For this review, take the finished solid that the model builds, in its own axes (mm). A direction names the side the tool comes from. Coordinates: 2 decimals unless noted, no trailing zeros. Loops run counter-clockwise (first coordinate to the right, second up) from the corner with the lowest first, then second, coordinate; pieces in that order, holes last. Notation, with made-up numbers: (48, 55) -> (103, 55) arc R24 ccw to (103, 86) -> close; hole circle Ø11 at (11.25, 42.5). An arc over 180 degrees is marked (long way). One line per item, written item: value.
from build123d import *

# Parameters (mm, degrees)
SKETCH1_W             = 38.1
SKETCH1_H             = 38.1
BOSS_EXTRUDE1_DEPTH   = 6.35
BOSS_EXTRUDE2_DEPTH   = 38.1
CUT_EXTRUDE1_DEPTH    = 39.1
F_4_CLEARANCE_HOLE1_D = 3.4544
SKETCH6_R             = 3.96875
CUT_EXTRUDE2_DEPTH    = 6.35


with BuildPart() as part:
    # Sketch1 → Boss-Extrude1 (new body)
    with BuildSketch(Plane(origin=(0, 0, 0), x_dir=(1, 0, 0), z_dir=(0, 1, 0))):
        Rectangle(SKETCH1_W, SKETCH1_H)
    extrude(amount=BOSS_EXTRUDE1_DEPTH)

    # Sketch2 → Boss-Extrude2 (add)
    with BuildSketch(Plane.XY.offset(19.05)):
        with BuildLine():
            Line((-19.05, 6.35), (19.05, 6.35))
            ThreePointArc((19.05, 6.35), (10.069743762, 10.06974368), (6.349999801, 19.049999801))
            Line((6.349999801, 19.049999801), (-6.350000199, 19.049999801))
            ThreePointArc((-6.350000199, 19.049999801), (-10.06974402, 10.069743821), (-19.05, 6.35))
        make_face()
    extrude(amount=-BOSS_EXTRUDE2_DEPTH)

    # Sketch3 → Cut-Extrude1 (cut, through all)
    with BuildSketch(Plane(origin=(19.05, 0, 0), x_dir=(0, 0, -1), z_dir=(1, 0, 0))):
        with BuildLine():
            Line((-19.05, 6.35), (-19.05, 19.049999801))
            Line((-19.05, 19.049999801), (-6.350000199, 19.049999801))
            ThreePointArc((-6.350000199, 19.049999801), (-10.06974402, 10.069743821), (-19.05, 6.35))
        make_face()
        with BuildLine():
            Line((19.05, 6.35), (19.05, 19.049999801))
            Line((19.05, 19.049999801), (6.350000199, 19.049999801))
            ThreePointArc((6.350000199, 19.049999801), (10.06974402, 10.069743821), (19.05, 6.35))
        make_face()
    extrude(amount=-CUT_EXTRUDE1_DEPTH, mode=Mode.SUBTRACT)

    # #4 Clearance Hole1 (through all)
    with Locations(Plane(origin=(0, 19.049999801, 0), x_dir=(1, 0, 0), z_dir=(0, 1, 0))):
        with Locations((0, 0)):
            Hole(F_4_CLEARANCE_HOLE1_D / 2)

    # Sketch6 → Cut-Extrude2 (cut)
    with BuildSketch(Plane.XZ):
        Circle(SKETCH6_R)
    extrude(amount=-CUT_EXTRUDE2_DEPTH, mode=Mode.SUBTRACT)


solid = part.part
1. Take a section at C-C, the plane y = 4. Give the boundary of the cut face in (x, z).
Return value:
outline: (-19.05, -19.05) -> (19.05, -19.05) -> (19.05, 19.05) -> (-19.05, 19.05) -> close; hole circle Ø7.94 at (0, 0)
2. Insertion check: pin 1 Ø6 at (x, z) = (-13.5, -11.5) entering from +Y; pin 2 Ø6 at (x, y) = (2, 16.5) entering from +Z; pin 3 Ø10 at (x, y) = (9, 12.5) entering from -Z. Each pin has a flat end and moves straight along its axis. Give the tip position at first contact, or say it passes through.
Return value:
pin 1: stops at y = 9.54
pin 2: stops at z = 7.63
pin 3: stops at z = -13.77
3. To check wall thickness, follow probe 1 along Z at (x, y) = (1, 14.75); probe 2 along Z at (x, y) = (0, 11.25); probe 3 along X at (y, z) = (12.75, 2). State the ranges of each line that lie inside material, in increasing order. Write a range as from..to.
Return value:
probe 1: z = -7.1..-1.41, 1.41..7.1
probe 2: z = -9.03..-1.73, 1.73..9.03
probe 3: x = -8.02..8.02
4. For faces 5 (the cylindrical face through (-0.86, 3.131, -3.874)), 6 (the cylindrical face through (-11.65, 8.73, 0.27)), list the 3-axis set-ups (+Z, -Z, +X, -X, +Y, -Y) from which the entire face can be reached by the end or side of a thin tool; tool diameter is ignored.
Return value:
face 5: -Y
face 6: +Z, -Z, -X, +Y
5. Take a section at A-A, the plane x = 0. Give the boundary of the cut face in (y, z), and give its area (3 significant figures).
Return value:
outline: (0, -19.05) -> (6.35, -19.05) arc R12.7 cw to (19.05, -6.35) -> (19.05, -1.73) -> (6.35, -1.73) -> (6.35, -3.97) -> (0, -3.97) -> close; (0, 3.97) -> (6.35, 3.97) -> (6.35, 1.73) -> (19.05, 1.73) -> (19.05, 6.35) arc R12.7 cw to (6.35, 19.05) -> (0, 19.05) -> close
area: 378 mm2
6. Take a section at D-D, the plane z = -12. Give the boundary of the cut face in (x, y).
Return value:
outline: (-19.05, 0) -> (19.05, 0) -> (19.05, 6.35) arc R12.7 cw to (12, 8.49) -> (-12, 8.49) arc R12.7 cw to (-19.05, 6.35) -> close
7. The part is to be moulded in two halves that separate along Z. For faces 1 (the flat face through (-19.05, 3, 0)), 2 (the flat face through (2, 6.35, -1)), 3 (the cylindrical face through (0.27, 8.73, 11.65)), 4 (the cylindrical face through (0.27, 8.73, -11.65)), say which applies: pulls with the +Z half, pulls with the -Z half, needs draft (parallel to the pull), parting line crosses it, or undercut.
Return value:
face 1: needs draft
face 2: undercut
face 3: pulls with the +Z half
face 4: pulls with the -Z half
8. Take a section at B-B, the plane z = 0. Give the boundary of the cut face in (x, y).
Return value:
outline: (-19.05, 0) -> (-3.97, 0) -> (-3.97, 6.35) -> (-1.73, 6.35) -> (-1.73, 19.05) -> (-6.35, 19.05) arc R12.7 cw to (-19.05, 6.35) -> close; (1.73, 6.35) -> (3.97, 6.35) -> (3.97, 0) -> (19.05, 0) -> (19.05, 6.35) arc R12.7 cw to (6.35, 19.05) -> (1.73, 19.05) -> close
